Verification items for this drawing (mm, ordinates from the low corner). A direction names the side the tool comes from. Round coordinates to 2 decimals unless told otherwise and drop trailing zeros. Order: outer loops, then holes, each group sorted by start corner. A loop starts at its lowest first (then second) coordinate and runs counter-clockwise, first axis right, second up. Notation, with made-up numbers: (72, 20.5) -> (76, 20.5) arc R21 cw to (76, 36.5) -> close; hole circle Ø1 at (-14.5, 13.25). An arc over 180 degrees is marked (long way). Answer in a Markdown table with one row per item. Add a question column.
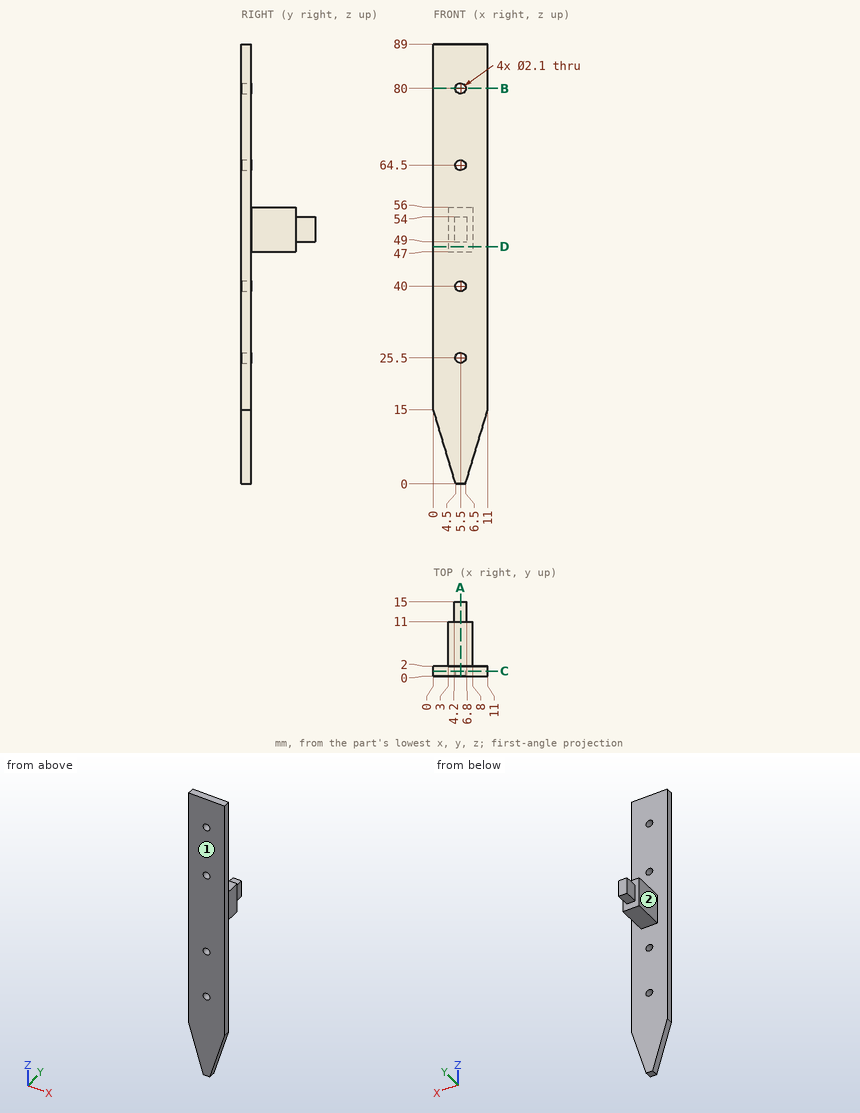
1) Thickness scan on L1, parallel to Z at x = 5.5, y = 0.45; L2, parallel to X at y = 0.7, z = 25.5; L3, parallel to Z at x = 7, y = 9.5. Record the ranges inside material, lowest first. Write a range as [from, to].
2) Cross-section at D-D, the plane z = 48. Record the boundary of the cut face in (x, y).
3) Cross-section at B-B, the plane z = 80. Record the boundary of the cut face in (x, y), and give its area (3 significant figures).
4) Tool access check on the marked faces 1 and 2. Record the directions out of +Z, -Z, +X, -X, +Y, -Y that give a thin tool (end or side, any length) a straight path to the whole face; none if there is none.
5) Cross-section at A-A, the plane x = 5.5. Record the boundary of the cut face in (y, z).
6) Depth check by flat-ended pin: P1, Ø1, axis at x = 3.5, y = 6, coming from the -Z side; P2, Ø2.5, axis at x = 5.5, z = 40, coming from the +Y side; P3, Ø2, axis at y = 7, z = 56.5, coming from the -X side. Enter the tip coordinate at first touch or a pass-through.
7) Cross-section at C-C, the plane y = 1. Record the boundary of the cut face in (x, z).
Results below:
| question | item | result |
|---|---|---|
| 1 | L1 | [0, 24.45], [26.55, 38.95], [41.05, 63.45], [65.55, 78.95], [81.05, 89] |
| 1 | L2 | [0, 4.45], [6.55, 11] |
| 1 | L3 | [47, 56] |
| 2 | outline | (0, 0) -> (11, 0) -> (11, 2) -> (8, 2) -> (8, 11) -> (3, 11) -> (3, 2) -> (0, 2) -> close |
| 3 | outline | (0, 0) -> (4.45, 0) -> (4.45, 2) -> (0, 2) -> close; (6.55, 0) -> (11, 0) -> (11, 2) -> (6.55, 2) -> close |
| 3 | area | 17.8 mm² |
| 4 | face 1 | +Z, -Z, +X, -X, -Y |
| 4 | face 2 | +Z, -Z, -X, +Y |
| 5 | outline | (0, 0) -> (2, 0) -> (2, 24.45) -> (0, 24.45) -> close; (0, 26.55) -> (2, 26.55) -> (2, 38.95) -> (0, 38.95) -> close; (0, 41.05) -> (2, 41.05) -> (2, 47) -> (11, 47) -> (11, 49) -> (15, 49) -> (15, 54) -> (11, 54) -> (11, 56) -> (2, 56) -> (2, 63.45) -> (0, 63.45) -> close; (0, 65.55) -> (2, 65.55) -> (2, 78.95) -> (0, 78.95) -> close; (0, 81.05) -> (2, 81.05) -> (2, 89) -> (0, 89) -> close |
| 6 | P1 | z = 47 |
| 6 | P2 | y = 2 |
| 6 | P3 | x = 3 |
| 7 | outline | (0, 15) -> (4.5, 0) -> (6.5, 0) -> (11, 15) -> (11, 89) -> (0, 89) -> close; hole circle Ø2.1 at (5.5, 25.5); hole circle Ø2.1 at (5.5, 40); hole circle Ø2.1 at (5.5, 64.5); hole circle Ø2.1 at (5.5, 80) |
